Geometry: see drawing. Coordinates: mm, zero at the bounding-box minimum. A direction names the side the tool comes from. Give positions to 0.01 mm unless a question says otherwise; leave off trailing zeros. Write each loop counter-clockwise with the first axis right and the second up, starting at its lowest first coordinate (ties: lowest second). Pieces come first, ordered by that corner, then holes. Notation, with made-up numbers: M 51.5,30.25 L 81.5,30.25 A21 cw 81.5,44.25 Z; hole C 88,-30 d2. An arc over 180 degrees is marked long. Answer as a JSON object with one key per item and string values. Group by question number.
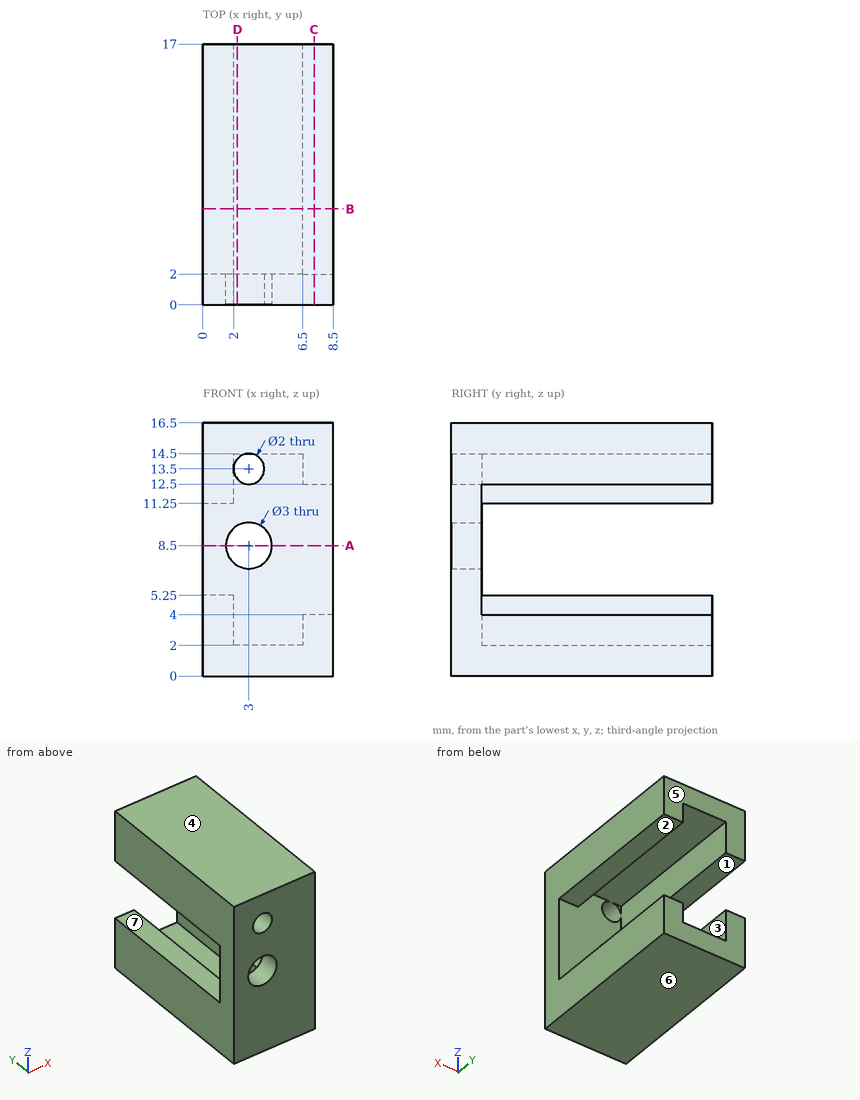
(1) Pull-direction query (Z, two-part tool) for the marked faces 4, 5, 6 and 7; classes: pulls with the +Z half, pulls with the -Z half, needs draft (parallel to the pull), parting line crosses it, or undercut.
(2) Access query for the marked faces 1, 2 and 3. Directions: +Z, -Z, +X, -X, +Y, -Y. A direction counts if a zero-diameter tool reaches every point of the face in a straight line with its end or side. Return the directions, or none.
(3) Section C-C, the plane x = 7.25. Return loops of the section in (y, z), plus the area to 3 significant figures.
(4) Section D-D, the plane x = 2.25. Return loops of the section in (y, z), plus the area to 3 significant figures.
(5) Contact query for flat-ended pins moving along their axis: pin 1 Ø3 at (x, z) = (5, 11) entering from +Y; pin 2 Ø1.6 at (x, z) = (3, 13.5) entering from +Y. Output: stop coordinate, or through.
(6) Section B-B, the plane y = 6.25. Return loops of the section in (x, z).
(7) Ray query, L1, parallel to Z at x = 3, y = 0.55; L2, parallel to Z at x = 3.75, y = 11.25; L3, parallel to Z at x = 7.75, y = 14.5. Return the intervals inside material, ascending. Write a range as [from, to].
(8) Section A-A, the plane z = 8.5. Return loops of the section in (x, y), plus the area to 3 significant figures.
Reported:
{
 "1": {"face 4": "pulls with the +Z half", "face 5": "needs draft", "face 6": "pulls with the -Z half", "face 7": "undercut"},
 "2": {"face 1": "+X, -X, +Y", "face 2": "+X, +Y", "face 3": "+Y"},
 "3": {"outline": "M 0,0 L 17,0 L 17,4 L 2,4 L 2,12.5 L 17,12.5 L 17,16.5 L 0,16.5 Z", "area": "153 mm2"},
 "4": {"outline": "M 0,0 L 17,0 L 17,2 L 2,2 L 2,7.2 L 0,7.2 Z; M 0,9.8 L 2,9.8 L 2,12.84 L 0,12.84 Z; M 0,14.16 L 2,14.16 L 2,14.5 L 17,14.5 L 17,16.5 L 0,16.5 Z", "area": "85.2 mm2"},
 "5": {"pin 1": "stops at y = 2", "pin 2": "passes through"},
 "6": {"outline": "M 0,0 L 8.5,0 L 8.5,4 L 6.5,4 L 6.5,2 L 2,2 L 2,5.25 L 0,5.25 Z; M 0,11.25 L 2,11.25 L 2,14.5 L 6.5,14.5 L 6.5,12.5 L 8.5,12.5 L 8.5,16.5 L 0,16.5 Z"},
 "7": {"L1": "z = [0, 7], [10, 12.5], [14.5, 16.5]", "L2": "z = [0, 2], [14.5, 16.5]", "L3": "z = [0, 4], [12.5, 16.5]"},
 "8": {"outline": "M 0,0 L 1.5,0 L 1.5,2 L 0,2 Z; M 4.5,0 L 8.5,0 L 8.5,2 L 4.5,2 Z", "area": "11.0 mm2"}
}
